```python
from build123d import *

# Parameters (mm, degrees)
BOSS_EXTRUDE7_DEPTH     = 10
SKETCH1_9_R             = 1
CUT_EXTRUDE4_DEPTH      = 19
CHAMFER1_SIZE           = 1
BOSS_EXTRUDE8_DEPTH     = 30
CUT_EXTRUDE7_DEPTH      = 42
CUT_EXTRUDE7_DEPTH_BACK = 39
SKETCH8_W               = 6
SKETCH8_H               = 15
SKETCH8_4_R             = 8.5
CUT_EXTRUDE8_DEPTH      = 24
CUT_EXTRUDE9_DEPTH      = 24
SKETCH10_R              = 1.375
CUT_EXTRUDE10_DEPTH     = 7
FILLET1_R               = 10


with BuildPart() as part:
    # Sketch1 → Boss-Extrude7 (new body)
    with BuildSketch(Plane.XY):
        Polygon((-34.62989834, 81.220503206), (4.762411781, 88.166430312), (18.654265994, 9.381810071), (-20.738044126, 2.435882965), align=None)
    extrude(amount=BOSS_EXTRUDE7_DEPTH)

    # Sketch1_9 → Cut-Extrude4 (cut)
    with BuildSketch(Plane.XY):
        with Locations(Location((-20.553187739, 71.088441211, 0), (0, 0, 180))):
            Circle(SKETCH1_9_R)
        with Locations(Location((-5, 73.830887845, 0), (0, 0, 180))):
            Circle(SKETCH1_9_R)
        with Locations(Location((-18.886713057, 65.324513545, 0), (0, 0, 180))):
            Circle(SKETCH1_9_R)
        with Locations(Location((-4.594594595, 67.844599641, 0), (0, 0, 180))):
            Circle(SKETCH1_9_R)
        with Locations(Location((-12.849965147, 72.875773723, 0), (0, 0, 180))):
            Circle(SKETCH1_9_R)
        with Locations(Location((-11.808076081, 66.966927205, 0), (0, 0, 180))):
            Circle(SKETCH1_9_R)
    extrude(amount=CUT_EXTRUDE4_DEPTH, mode=Mode.SUBTRACT)

    # Chamfer1
    chamfer1_edges = [part.edges().sort_by_distance(p)[0] for p in [
        (-4, 73.830887845, 10),
        (-3.594594595, 67.844599641, 10),
        (-17.886713057, 65.324513545, 10),
        (-11.849965147, 72.875773723, 10),
        (-10.808076081, 66.966927205, 10),
        (-19.553187739, 71.088441211, 10),
    ]]
    chamfer(chamfer1_edges, length=CHAMFER1_SIZE)

    # Sketch6 → Boss-Extrude8 (add)
    with BuildSketch(Plane.XY.offset(10)):
        Polygon((-30.288693898, 56.60030938), (-27.683971233, 41.828193085), (11.708338888, 48.774120192), (9.103616223, 63.546236487), align=None)
        Polygon((16.049543329, 24.153926367), (-23.342766791, 17.20799926), (-20.738044126, 2.435882965), (18.654265994, 9.381810071), align=None)
    extrude(amount=BOSS_EXTRUDE8_DEPTH)

    # Sketch8 → Cut-Extrude7 (cut, two sides: drawn at the far end of the back side and taken through both)
    with BuildSketch(Plane(origin=(-3.646611731, 20.680962813, 0), x_dir=(0.984807753012227, 0.1736481776668232, 0), z_dir=(-0.1736481776668232, 0.984807753012227, 0)).offset(-CUT_EXTRUDE7_DEPTH_BACK)):
        Polygon((-20, -25), (-14, -25), (-20, -10), align=None)
        with Locations((-17, -32.5)):
            Rectangle(SKETCH8_W, SKETCH8_H)
        with Locations((17, -32.5)):
            Rectangle(SKETCH8_W, SKETCH8_H)
        Polygon((20, -10), (14, -25), (20, -25), align=None)
    extrude(amount=CUT_EXTRUDE7_DEPTH + CUT_EXTRUDE7_DEPTH_BACK, mode=Mode.SUBTRACT)

    # Sketch8_4 → Cut-Extrude8 (cut)
    with BuildSketch(Plane(origin=(-3.646611731, 20.680962813, 0), x_dir=(0.984807753012227, 0.1736481776668232, 0), z_dir=(-0.1736481776668232, 0.984807753012227, 0))):
        with Locations((0, -25)):
            Circle(SKETCH8_4_R)
        with BuildLine():
            ThreePointArc((8.5, -25), (0, -33.5), (-8.5, -25))
            Line((-8.5, -25), (-14, -25))
            Line((-14, -25), (-14, -40))
            Line((-14, -40), (14, -40))
            Line((14, -40), (14, -25))
            Line((14, -25), (8.5, -25))
        make_face()
    extrude(amount=-CUT_EXTRUDE8_DEPTH, mode=Mode.SUBTRACT)

    # Sketch7 → Cut-Extrude9 (cut)
    with BuildSketch(Plane(origin=(-10.592538838, 60.073272934, 0), x_dir=(0.984807753012227, 0.17364817766682317, 0), z_dir=(-0.17364817766682317, 0.984807753012227, 0))):
        Polygon((-14, -25), (-20, -10), (-20, -40), (-8, -40), align=None)
        with BuildLine():
            Line((8, -40), (14, -25))
            Line((14, -25), (7, -25))
            ThreePointArc((7, -25), (0, -32), (-7, -25))
            Line((-7, -25), (-14, -25))
            Line((-14, -25), (-8, -40))
            Line((-8, -40), (8, -40))
        make_face()
        Polygon((20, -40), (20, -10), (14, -25), (8, -40), align=None)
        with BuildLine():
            ThreePointArc((-7, -25), (0, -32), (7, -25))
            Line((7, -25), (-7, -25))
        make_face()
        with BuildLine():
            Line((-7, -25), (7, -25))
            ThreePointArc((7, -25), (0, -18), (-7, -25))
        make_face()
    extrude(amount=-CUT_EXTRUDE9_DEPTH, mode=Mode.SUBTRACT)

    # Sketch10 → Cut-Extrude10 (cut)
    with BuildSketch(Plane.XY.offset(25)):
        with Locations((-13.42333762, 11.341362667)):
            Circle(SKETCH10_R)
        with Locations((8.734836823, 15.248446664)):
            Circle(SKETCH10_R)
        with Locations((-20.369264727, 50.733672787)):
            Circle(SKETCH10_R)
        with Locations((1.788909716, 54.640756785)):
            Circle(SKETCH10_R)
    extrude(amount=-CUT_EXTRUDE10_DEPTH, mode=Mode.SUBTRACT)

    # Fillet1
    fillet1_edges = [part.edges().sort_by_distance(p)[0] for p in [
        (-34.62989834, 81.220503206, 5),
        (4.762411781, 88.166430312, 5),
    ]]
    fillet(fillet1_edges, radius=FILLET1_R)


solid = part.part
```
Could you check a few things on this model? Use its own coordinates, in mm. A direction names the side the tool comes from. Round coordinates to 2 decimals unless told otherwise and drop trailing zeros. Order: outer loops, then holes, each group sorted by start corner. A loop starts at its lowest first (then second) coordinate and runs counter-clockwise, first axis right, second up. Notation, with made-up numbers: M 14,63 L 28,63 A17 cw 28,81 Z; hole C 47,41 d11. An arc over 180 degrees is marked long. One line per question, with ' | ' between items. Start each with the question number.
(1) Suppose I cut it at B-B on z = 14.5. List the corners of the cut face in (x, y) for me, then the cut area to 3 significant figures.
(2) For faces 1 (the face through (-7, 45, 0)), 2 (the face through (8.437, 13.906, 21.549)), which set-ups out of +Z, -Z, +X, -X, +Y, -Y let a thin tool reach every point of the face, with its end or its side?
(3) Please list where these lines run through material, in increasing order: line 1 along Z through (x, y) = (-9.5, 43.5); line 2 along Y through (x, z) = (-13.5, 21.5); line 3 along Y through (x, z) = (-11.5, 7.5).
(4) Thinking about a two-plate mould opening in Y: for faces 3 (the face through (-13, 11, 18)), 4 (the face through (14.457, 16.151, 17.395)), 5 (the face through (-18.8, 51.1, 25)), 6 (the face through (-3.37, 20.73, 15.73)), which applies, +Y half, -Y half, draft (parallel to the pull), parting line (faces both ways), or undercut?
(5) Suppose I cut it at A-A on z = 4.5. List the corners of the cut face in (x, y) for me.
(6) For P1, Ø2.5, axis at x = -11.81, y = 66.97, coming from the +Z side; P2, Ø1.4, axis at x = -13.5, y = 11.5, coming from the +Z side; P3, Ø10, axis at y = 70.5, z = 10.5, coming from the +X side; P4, Ø1.2, axis at x = -4.59, y = 67.84, coming from the -Z side, each with a flat end and sliding along its axis, tell me the tip position at first contact or that it passes through.
(7) Suppose I cut it at C-C on y = 39. List the corners of the cut face in (x, z) for me.
Geometry results:
1) outline: M -28.52,56.91 L -25.91,42.14 L 9.94,48.46 L 7.33,63.23 Z; M -21.57,17.52 L -18.97,2.75 L 16.88,9.07 L 14.28,23.84 Z | area: 1,090 mm²
2) face 1: -Z, +X, -X, +Y, -Y | face 2: +Z
3) line 1: 0 to 10 | line 2: 3.71 to 9.97, 12.71 to 18.94 | line 3: 4.06 to 66.02, 67.92 to 85.3
4) face 3: undercut | face 4: +Y half | face 5: draft | face 6: undercut
5) outline: M -32.89,71.37 L -20.74,2.44 L 18.65,9.38 L 6.5,78.32 A10 ccw -5.09,86.43 L -24.78,82.96 A10 ccw Z; hole C -20.55,71.09 d2; hole C -18.89,65.32 d2; hole C -12.85,72.88 d2; hole C -11.81,66.97 d2; hole C -5,73.83 d2; hole C -4.59,67.84 d2
6) P1: z = 9.25 | P2: z = 18 | P3: x = 8.75 | P4: through
7) outline: M -27.19,0 L 13.43,0 L 13.43,10 L -27.19,10 Z
